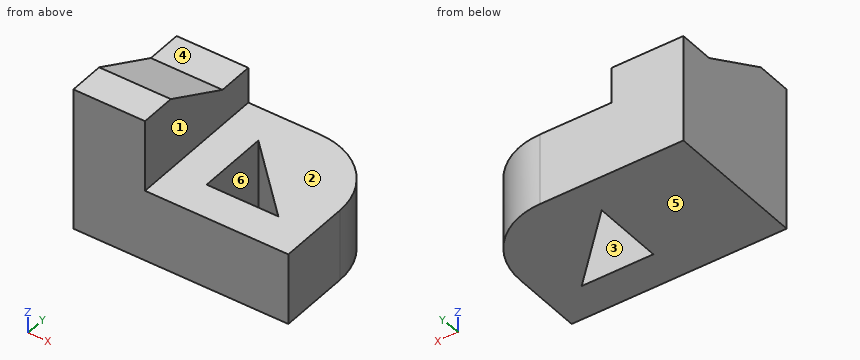
```python
from build123d import *

# Parameters (mm, degrees)
F1_DEPTH = 20
F3_DEPTH = 20.001
F5_DEPTH = 20


with BuildPart() as f1:
    # F0 (on Top) → F1 (new body)
    with BuildSketch(Plane.XY):
        with BuildLine():
            Line((0, 40), (0, 0))
            Line((0, 0), (60, 0))
            Line((60, 0), (60, 20))
            ThreePointArc((60, 20), (54.142136, 34.142136), (40, 40))
            Line((40, 40), (0, 40))
        make_face()
    extrude(amount=F1_DEPTH)

    # F2 (on face) → F3 (cut, through all)
    with BuildSketch(Plane.XY.offset(20)):
        Polygon((50, 10), (30, 30), (30, 10), align=None)
    extrude(amount=-F3_DEPTH, mode=Mode.SUBTRACT)

    # F4 (on Right) → F5 (join)
    with BuildSketch(Plane.YZ):
        Polygon((0, 40), (0, 20), (40, 20), (40, 30), (30, 30), (10, 40), align=None)
    extrude(amount=F5_DEPTH)


solid = f1.part
```
Here's how the part is built. I have some questions about the finished solid (model axes, mm). Face numbers are marked on the shaded views. A direction names the side the tool comes from. Round coordinates to 2 decimals unless told otherwise and drop trailing zeros. Order: outer loops, then holes, each group sorted by start corner. A loop starts at its lowest first (then second) coordinate and runs counter-clockwise, first axis right, second up. Notation, with made-up numbers: M 25.25,67.25 L 56.25,67.25 A21 cw 56.25,82.25 Z; hole C 30.5,36.25 d6. An arc over 180 degrees is marked long. Answer in a Markdown table with one row per item.
Item 1: Imagine slicing it at A-A, the plane x = 32.5. Write out the boundary of the cut face in (y, z), and give its area (3 significant figures).
A:
| item | result |
|---|---|
| outline | M 0,0 L 10,0 L 10,20 L 0,20 Z; M 27.5,0 L 40,0 L 40,20 L 27.5,20 Z |
| area | 450 mm2 |
Item 2: I'm going to push flat-ended pins straight in: pin 1 (4 mm diameter, centred on x = 46.5, y = 28.5, fed in from +Z); pin 2 (6 mm diameter, centred on y = 13.5, z = 26.5, fed in from +X); pin 3 (3 mm diameter, centred on x = 14, y = 35, fed in from +Z). Where does each tip first touch, or does it pass through?
A:
| item | result |
|---|---|
| pin 1 | stops at z = 20 |
| pin 2 | stops at x = 20 |
| pin 3 | stops at z = 30 |
Item 3: Thinking about a two-plate mould opening in X: for the marked faces 1, 2 and 3, which applies, +X half, -X half, draft (parallel to the pull), parting line (faces both ways), or undercut?
A:
| item | result |
|---|---|
| face 1 | +X half |
| face 2 | draft |
| face 3 | undercut |
Item 4: If I drill on L1, parallel to Z at x = 47, y = 31; L2, parallel to Y at x = 40, z = 2, over which ranges is the centre line in solid material (lowest first)? Write a range as from..to.
A:
| item | result |
|---|---|
| L1 | z = 0..20 |
| L2 | y = 0..10, 20..40 |
Item 5: Imagine slicing it at C-C, the plane z = 15. Write out the boundary of the cut face in (x, y).
A:
| item | result |
|---|---|
| outline | M 0,0 L 60,0 L 60,20 A20 ccw 40,40 L 0,40 Z; hole M 30,10 L 50,10 L 30,30 Z |
Item 6: Imagine slicing it at B-B, the plane y = 16. Write out the boundary of the cut face in (x, z), and give its area (3 significant figures).
A:
| item | result |
|---|---|
| outline | M 0,0 L 30,0 L 30,20 L 20,20 L 20,37 L 0,37 Z; M 44,0 L 60,0 L 60,20 L 44,20 Z |
| area | 1,260 mm2 |
Item 7: For the marked faces 4, 5 and 6, which set-ups out of +Z, -Z, +X, -X, +Y, -Y let a thin tool reach every point of the face, with its end or its side?
A:
| item | result |
|---|---|
| face 4 | +Z, +X, -X, +Y |
| face 5 | -Z, +X, -X, +Y, -Y |
| face 6 | +Z, -Z |
Item 8: Imagine slicing it at D-D, the plane x = 13. Write out the boundary of the cut face in (y, z), and give its area (3 significant figures).
A:
| item | result |
|---|---|
| outline | M 0,0 L 40,0 L 40,30 L 30,30 L 10,40 L 0,40 Z |
| area | 1,400 mm2 |
